from build123d import *

# Parameters (mm, degrees)
BOX_EXTRUDE_DEPTH                 = 12.5
SHELL1_T                          = -3
CUT_SWEEP_START                   = -12.5
CUT_SWEEP_DEPTH                   = 4.5
SKETCH2_W                         = 10
SKETCH2_H                         = 10
SQUARES_EXTRUDE_DEPTH             = 9.5
SKETCH11_W                        = 10
SKETCH11_H                        = 31
SKETCH11_W_2                      = 31
SKETCH11_H_2                      = 10
CUT_EXTRUDE2_DEPTH                = 264.732611064
SQUARES_M3_CLEARANCE_HOLES_D      = 2.5
SQUARES_M3_CLEARANCE_HOLES_DEPTH  = 2
SQUARES_M3_CLEARANCE_HOLES_TIP    = 0.751075774
F_8_0MM_DOWEL_HOLE1_D             = 8
F_8_0MM_DOWEL_HOLE1_DEPTH         = 7.5
F_8_0MM_DOWEL_HOLE1_TIP           = 2.403442476
F_5_0MM_DOWEL_HOLE1_D             = 5
F_5_0MM_DOWEL_HOLE1_DEPTH         = 7.5
F_5_0MM_DOWEL_HOLE1_TIP           = 1.502151548
M3_CLEARANCE_HOLE3_D              = 3.4
M3_CLEARANCE_HOLE3_DEPTH          = 7.5
M3_CLEARANCE_HOLE3_TIP            = 1.021463052
M3X0_5_TAPPED_HOLE1_D             = 2.5
M3X0_5_TAPPED_HOLE2_D             = 2.5
M3X0_5_TAPPED_HOLE2_DEPTH         = 7.5
M3X0_5_TAPPED_HOLE2_TIP           = 0.751075774
SKETCH25_W                        = 3
SKETCH25_H                        = 31
SKETCH25_W_2                      = 31
SKETCH25_H_2                      = 3
DRIVER_BOARD_HOLDER_EXTRUDE_DEPTH = 38.75
F_2_5MM_DOWEL_HOLE1_D             = 2.5
F_2_5MM_DOWEL_HOLE1_ON_FACE_2_D   = 2.5


# Read off the part's stored shape, not the designer's step: Cut-Sweep
with BuildPart() as part:
    # Sketch1 → Box-Extrude (new body)
    with BuildSketch(Plane.XY):
        with BuildLine():
            Line((-54.633571826, -76.683344949), (169.366428174, -76.683344949))
            ThreePointArc((169.366428174, -76.683344949), (183.508563798, -70.825480573), (189.366428174, -56.683344949))
            Line((189.366428174, -56.683344949), (189.366428174, 163.316655051))
            ThreePointArc((189.366428174, 163.316655051), (183.508563798, 177.458790675), (169.366428174, 183.316655051))
            Line((169.366428174, 183.316655051), (139.366428174, 183.316655051))
            ThreePointArc((139.366428174, 183.316655051), (125.22429255, 177.458790675), (119.366428174, 163.316655051))
            Line((119.366428174, 163.316655051), (119.366428174, 33.316655051))
            ThreePointArc((119.366428174, 33.316655051), (113.508563798, 19.174519427), (99.366428174, 13.316655051))
            Line((99.366428174, 13.316655051), (-54.633571826, 13.316655051))
            ThreePointArc((-54.633571826, 13.316655051), (-68.77570745, 7.458790675), (-74.633571826, -6.683344949))
            Line((-74.633571826, -6.683344949), (-74.633571826, -56.683344949))
            ThreePointArc((-74.633571826, -56.683344949), (-68.77570745, -70.825480573), (-54.633571826, -76.683344949))
        make_face()
    extrude(amount=-BOX_EXTRUDE_DEPTH)

    # Shell1
    shell1_openings = [part.faces().sort_by_distance(p)[0] for p in [
        (90.029023859, 11.315684384, -12.5),
    ]]
    offset(amount=SHELL1_T, openings=shell1_openings, kind=Kind.INTERSECTION)

    # Cut-Sweep outline → Cut-Sweep (cut)
    with BuildSketch(Plane.XY.offset(CUT_SWEEP_START)):
        with BuildLine():
            Line((189.366428174, -56.683344949), (189.366428174, 163.316655051))
            ThreePointArc((189.366428174, 163.316655051), (183.508563798, 177.458790675), (169.366428174, 183.316655051))
            Line((169.366428174, 183.316655051), (139.366428174, 183.316655051))
            ThreePointArc((139.366428174, 183.316655051), (125.22429255, 177.458790675), (119.366428174, 163.316655051))
            Line((119.366428174, 163.316655051), (119.366428174, 33.316655051))
            ThreePointArc((119.366428174, 33.316655051), (113.508563798, 19.174519427), (99.366428174, 13.316655051))
            Line((99.366428174, 13.316655051), (-54.633571826, 13.316655051))
            ThreePointArc((-54.633571826, 13.316655051), (-68.77570745, 7.458790675), (-74.633571826, -6.683344949))
            Line((-74.633571826, -6.683344949), (-74.633571826, -56.683344949))
            ThreePointArc((-74.633571826, -56.683344949), (-68.77570745, -70.825480573), (-54.633571826, -76.683344949))
            Line((-54.633571826, -76.683344949), (169.366428174, -76.683344949))
            ThreePointArc((169.366428174, -76.683344949), (183.508563798, -70.825480573), (189.366428174, -56.683344949))
        make_face()
        with BuildLine():
            Line((169.366428174, -75.183344949), (-54.633571826, -75.183344949))
            ThreePointArc((-54.633571826, -75.183344949), (-67.715047278, -69.764820401), (-73.133571826, -56.683344949))
            Line((-73.133571826, -56.683344949), (-73.133571826, -6.683344949))
            ThreePointArc((-73.133571826, -6.683344949), (-67.715047278, 6.398130503), (-54.633571826, 11.816655051))
            Line((-54.633571826, 11.816655051), (99.366428174, 11.816655051))
            ThreePointArc((99.366428174, 11.816655051), (114.569223969, 18.113859256), (120.866428174, 33.316655051))
            Line((120.866428174, 33.316655051), (120.866428174, 163.316655051))
            ThreePointArc((120.866428174, 163.316655051), (126.284952722, 176.398130503), (139.366428174, 181.816655051))
            Line((139.366428174, 181.816655051), (169.366428174, 181.816655051))
            ThreePointArc((169.366428174, 181.816655051), (182.447903626, 176.398130503), (187.866428174, 163.316655051))
            Line((187.866428174, 163.316655051), (187.866428174, -56.683344949))
            ThreePointArc((187.866428174, -56.683344949), (182.447903626, -69.764820401), (169.366428174, -75.183344949))
        make_face(mode=Mode.SUBTRACT)
    extrude(amount=CUT_SWEEP_DEPTH, mode=Mode.SUBTRACT)

    # Sketch2 → Squares-Extrude (add)
    with BuildSketch(Plane.XY.offset(-3)):
        with Locations((41.816428174, 5.316655051)):
            Rectangle(SKETCH2_W, SKETCH2_H)
        with Locations((181.366428174, -33.683344949)):
            Rectangle(SKETCH2_W, SKETCH2_H)
        with Locations((41.366428174, -68.683344949)):
            Rectangle(SKETCH2_W, SKETCH2_H)
        with Locations((181.366428174, 140.316655051)):
            Rectangle(SKETCH2_W, SKETCH2_H)
    extrude(amount=-SQUARES_EXTRUDE_DEPTH)

    # Sketch11 → Cut-Extrude2 (cut, through all)
    with BuildSketch(Plane(origin=(0, 0, -3), x_dir=(-1, 0, 0), z_dir=(0, 0, -1))):
        with BuildLine():
            Line((-166.366428174, -44.683344949), (-110.366428174, -44.683344949))
            ThreePointArc((-110.366428174, -44.683344949), (-108.952214612, -44.097558511), (-108.366428174, -42.683344949))
            Line((-108.366428174, -42.683344949), (-108.366428174, -6.683344949))
            ThreePointArc((-108.366428174, -6.683344949), (-108.952214612, -5.269131386), (-110.366428174, -4.683344949))
            Line((-110.366428174, -4.683344949), (-166.366428174, -4.683344949))
            ThreePointArc((-166.366428174, -4.683344949), (-167.780641736, -5.269131386), (-168.366428174, -6.683344949))
            Line((-168.366428174, -6.683344949), (-168.366428174, -42.683344949))
            ThreePointArc((-168.366428174, -42.683344949), (-167.780641736, -44.097558511), (-166.366428174, -44.683344949))
        make_face()
        with Locations((62.633571826, -22.513344949)):
            Rectangle(SKETCH11_W, SKETCH11_H)
        with Locations((-152.479428174, 162.176655051)):
            Rectangle(SKETCH11_W_2, SKETCH11_H_2)
    extrude(amount=-CUT_EXTRUDE2_DEPTH, mode=Mode.SUBTRACT)

    # Squares M3 Clearance Holes
    with Locations(Plane(origin=(0, 0, -12.5), x_dir=(1, 0, 0), z_dir=(0, 0, -1))):
        with Locations((41.816428174, -5.316655051), (181.366428174, -140.316655051), (181.366428174, 33.683344949), (41.366428174, 68.683344949)):
            Hole(SQUARES_M3_CLEARANCE_HOLES_D / 2, depth=SQUARES_M3_CLEARANCE_HOLES_DEPTH)
            with Locations((0, 0, -(SQUARES_M3_CLEARANCE_HOLES_DEPTH + SQUARES_M3_CLEARANCE_HOLES_TIP / 2))):  # 118° drill point
                Cone(0, SQUARES_M3_CLEARANCE_HOLES_D / 2, SQUARES_M3_CLEARANCE_HOLES_TIP, mode=Mode.SUBTRACT)

    # Ø8.0mm Dowel Hole1
    with Locations(Plane(origin=(169.366428174, -63.683344949, -3), x_dir=(-1, 0, 0), z_dir=(0, 0, -1))):
        with Locations((0, 0), (31, 0), (62, 0), (71, 67), (-9, 67)):
            Hole(F_8_0MM_DOWEL_HOLE1_D / 2, depth=F_8_0MM_DOWEL_HOLE1_DEPTH)
            with Locations((0, 0, -(F_8_0MM_DOWEL_HOLE1_DEPTH + F_8_0MM_DOWEL_HOLE1_TIP / 2))):  # 118° drill point
                Cone(0, F_8_0MM_DOWEL_HOLE1_D / 2, F_8_0MM_DOWEL_HOLE1_TIP, mode=Mode.SUBTRACT)

    # Ø5.0mm Dowel Hole1
    with Locations(Plane(origin=(0, 0, -3), x_dir=(-1, 0, 0), z_dir=(0, 0, -1))):
        with Locations((-138.366428174, -0.683344949)):
            Hole(F_5_0MM_DOWEL_HOLE1_D / 2, depth=F_5_0MM_DOWEL_HOLE1_DEPTH)
            with Locations((0, 0, -(F_5_0MM_DOWEL_HOLE1_DEPTH + F_5_0MM_DOWEL_HOLE1_TIP / 2))):  # 118° drill point
                Cone(0, F_5_0MM_DOWEL_HOLE1_D / 2, F_5_0MM_DOWEL_HOLE1_TIP, mode=Mode.SUBTRACT)

    # M3 Clearance Hole3
    with Locations(Plane(origin=(0, 0, -3), x_dir=(-1, 0, 0), z_dir=(0, 0, -1))):
        with Locations((-163.366428174, 6.316655051), (-113.366428174, 6.316655051), (-163.366428174, -70.683344949), (-113.366428174, -70.683344949)):
            Hole(M3_CLEARANCE_HOLE3_D / 2, depth=M3_CLEARANCE_HOLE3_DEPTH)
            with Locations((0, 0, -(M3_CLEARANCE_HOLE3_DEPTH + M3_CLEARANCE_HOLE3_TIP / 2))):  # 118° drill point
                Cone(0, M3_CLEARANCE_HOLE3_D / 2, M3_CLEARANCE_HOLE3_TIP, mode=Mode.SUBTRACT)

    # M3x0.5 Tapped Hole1 (through all)
    with Locations(Plane(origin=(0, 0, -3), x_dir=(-1, 0, 0), z_dir=(0, 0, -1))):
        with Locations((-117.116428174, -48.423344949), (-159.616428174, -48.423344949), (-89.226428174, -3.763344949), (-89.226428174, -43.263344949), (-171.219428174, 10.316655051), (-131.719428174, 10.316655051)):
            Hole(M3X0_5_TAPPED_HOLE1_D / 2)

    # M3x0.5 Tapped Hole2
    with Locations(Plane.XY):
        with Locations((-66.633571826, -3.183344949), (-66.633571826, -60.183344949), (172.479428174, 175.316655051), (132.479428174, 175.316655051)):
            Hole(M3X0_5_TAPPED_HOLE2_D / 2, depth=M3X0_5_TAPPED_HOLE2_DEPTH)
            with Locations((0, 0, -(M3X0_5_TAPPED_HOLE2_DEPTH + M3X0_5_TAPPED_HOLE2_TIP / 2))):  # 118° drill point
                Cone(0, M3X0_5_TAPPED_HOLE2_D / 2, M3X0_5_TAPPED_HOLE2_TIP, mode=Mode.SUBTRACT)

    # Sketch25 → Driver Board holder Extrude (add)
    with BuildSketch(Plane(origin=(0, 0, -3), x_dir=(-1, 0, 0), z_dir=(0, 0, -1))):
        with Locations((56.133571826, -22.513344949)):
            Rectangle(SKETCH25_W, SKETCH25_H)
        with Locations((-152.479428174, 155.676655051)):
            Rectangle(SKETCH25_W_2, SKETCH25_H_2)
    extrude(amount=DRIVER_BOARD_HOLDER_EXTRUDE_DEPTH)

    # Ø2.5mm Dowel Hole1 (through all)
    with Locations(Plane(origin=(163.979428174, 154.176655051, -37.25), x_dir=(0, 0, -1), z_dir=(0, -1, 0))):
        with Locations((0, 0), (0, -23), (-23, 0), (-23, -23)):
            Hole(F_2_5MM_DOWEL_HOLE1_D / 2)

    # Ø2.5mm Dowel Hole1 on face 2 (through all)
    with Locations(Plane(origin=(-54.633571826, -11.013344949, -37.25), x_dir=(0, 0, 1), z_dir=(1, 0, 0))):
        with Locations((0, 0), (0, 23), (23, 23), (23, 0)):
            Hole(F_2_5MM_DOWEL_HOLE1_ON_FACE_2_D / 2)


solid = part.part
Here's how the part is built. I have some questions about the finished solid (model axes, mm). A direction names the side the tool comes from. Give positions to 0.01 mm unless a question says otherwise; leave off trailing zeros. Order: outer loops, then holes, each group sorted by start corner. A loop starts at its lowest first (then second) coordinate and runs counter-clockwise, first axis right, second up. Notation, with made-up numbers: M 62,57 L 73,57 A30 cw 73,82 Z; hole C 29,65 d11. An arc over 180 degrees is marked long. Answer as a JSON object with one key per item and string values. Group by question number.
1) I'm going to push flat-ended pins straight in: pin 1 Ø5 at (y, z) = (-28, -27) entering from -X; pin 2 Ø2.5 at (x, z) = (57.5, -2.5) entering from +Y; pin 3 Ø3.5 at (x, z) = (28.5, -10.5) entering from +Y; pin 4 Ø4 at (x, y) = (148, 23.5) entering from +Z. Where does each tip first touch, or does it pass through?
2) Suppose I cut it at C-C, the plane y = 118. Write out the boundary of the cut face in (x, z).
3) We'd pull the mould along Y, two halves only. Please class faces 1 (the cylindrical face through (113.66, 19.33, -3.94)), 2 (the flat face through (181, 145.317, -8)), 3 (the cylindrical face through (182.59, -69.62, -10.28)), 4 (the cylindrical face through (173.06, -65.22, -1.48)): pulls with the +Y half, pulls with the -Y half, needs draft (parallel to the pull), parting line crosses it, or undercut.
4) Suppose I cut it at A-A, the plane z = -23.5. Write out the boundary of the cut face in (x, y).
5) Please list where these lines run through material, in increasing order: L1, parallel to Y at x = -56, z = -37; L2, parallel to X at y = 156, z = -14; L3, parallel to X at y = 155.55, z = -37.25. Write a range as [from, to].
6) On a 3-axis mill with a long thin cutter (end or side, diameter ignored), from which of +Z, -Z, +X, -X, +Y, -Y can I reach the whole of each face in a straight line? I mean faces 5 (the flat face through (186.366, 154, -8)), 6 (the cylindrical face through (142.06, -65.22, -1.48)). Say none if no direction works.
7) Suppose I cut it at B-B, the plane x = 82. Write out the boundary of the cut face in (y, z).
Results found:
{
 "1": {"pin 1": "x = -57.63", "pin 2": "y = 13.32", "pin 3": "y = 11.82", "pin 4": "z = 0"},
 "2": {"outline": "M 119.37,-8 L 120.87,-8 L 120.87,-12.5 L 122.37,-12.5 L 122.37,-3 L 186.37,-3 L 186.37,-12.5 L 187.87,-12.5 L 187.87,-8 L 189.37,-8 L 189.37,0 L 119.37,0 Z"},
 "3": {"face 1": "pulls with the +Y half", "face 2": "undercut", "face 3": "pulls with the -Y half", "face 4": "undercut"},
 "4": {"outline": "M -57.63,-38.01 L -54.63,-38.01 L -54.63,-7.01 L -57.63,-7.01 Z; M 136.98,154.18 L 167.98,154.18 L 167.98,157.18 L 136.98,157.18 Z"},
 "5": {"L1": "[-38.01, -35.24], [-32.79, -12.24], [-9.79, -7.01]", "L2": "[136.98, 139.75], [142.2, 162.75], [165.2, 167.98]", "L3": "[136.98, 139.73], [142.23, 162.73], [165.23, 167.98]"},
 "6": {"face 5": "-Z", "face 6": "+Z, -Z"},
 "7": {"outline": "M -76.68,-8 L -75.18,-8 L -75.18,-12.5 L -73.68,-12.5 L -73.68,-3 L 10.32,-3 L 10.32,-12.5 L 11.82,-12.5 L 11.82,-8 L 13.32,-8 L 13.32,0 L -76.68,0 Z"}
}
